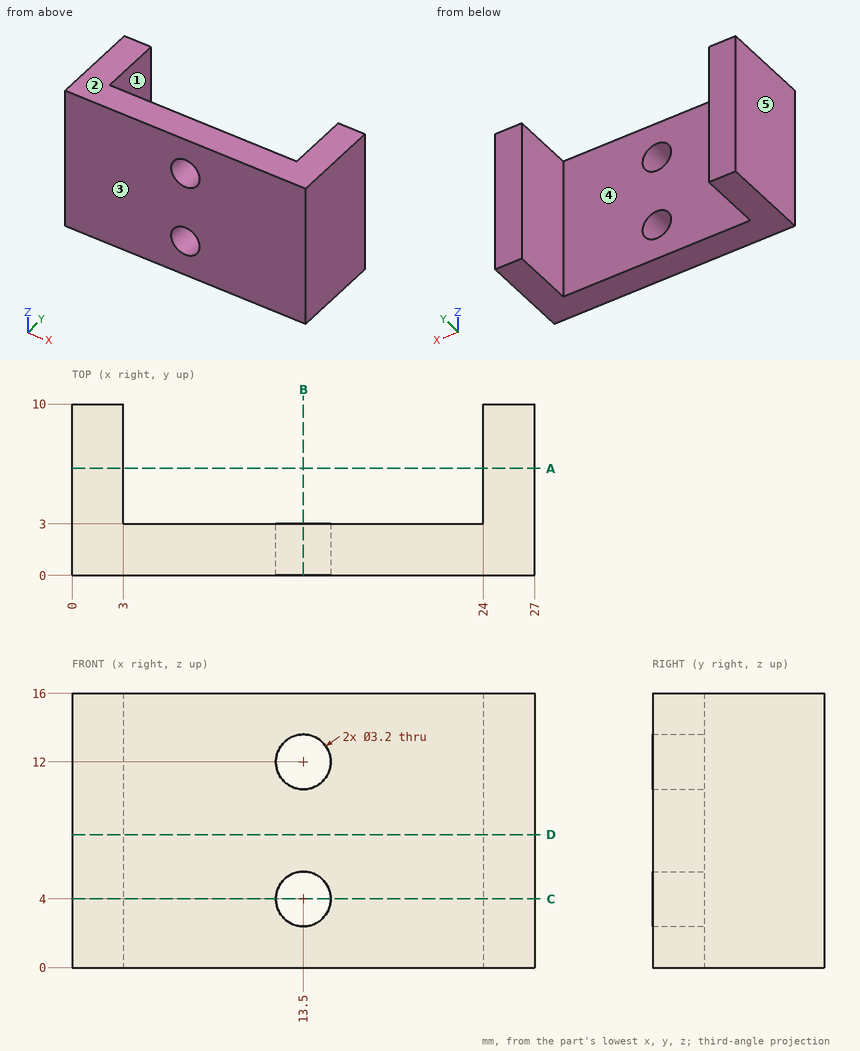
Job drawing, mm, ordinate dimensions from the low corner. One solid piece. A direction names the side the tool comes from. Round coordinates to 2 decimals unless told otherwise and drop trailing zeros. Order: outer loops, then holes, each group sorted by start corner. A loop starts at its lowest first (then second) coordinate and runs counter-clockwise, first axis right, second up. Notation, with made-up numbers: (76.5, 41) -> (132.5, 41) arc R33 ccw to (132.5, 80) -> close; hole circle Ø4 at (70, 31.25). An arc over 180 degrees is marked (long way). Answer in a Markdown table with one row per item.
1) Band-saw the part on A-A on y = 6.25. Give the cut face in (x, z), and give its area (3 significant figures).
Values:
| item | result |
|---|---|
| outline | (0, 0) -> (3, 0) -> (3, 16) -> (0, 16) -> close; (24, 0) -> (27, 0) -> (27, 16) -> (24, 16) -> close |
| area | 96.0 mm2 |
2) Mould opens along X. For the marked faces 3, 4 and 5 say: released by +X, released by -X, zero draft, split by the parting line, or undercut.
Values:
| item | result |
|---|---|
| face 3 | zero draft |
| face 4 | undercut |
| face 5 | released by -X |
3) Wall check: L1, parallel to Z at x = 13.5, y = 0.75; L2, parallel to X at y = 7.25, z = 7; L3, parallel to Y at x = 8, z = 1. Give the ranges that are in metal, low to high.
Values:
| item | result |
|---|---|
| L1 | 0 to 2.4, 5.6 to 10.4, 13.6 to 16 |
| L2 | 0 to 3, 24 to 27 |
| L3 | 0 to 3 |
4) Band-saw the part on D-D on z = 7.75. Give the cut face in (x, y).
Values:
| item | result |
|---|---|
| outline | (0, 0) -> (27, 0) -> (27, 10) -> (24, 10) -> (24, 3) -> (3, 3) -> (3, 10) -> (0, 10) -> close |
5) Pin check, flat tip, straight feed: P1, Ø5, axis at x = 13.5, z = 4, coming from the +Y side. Stop position of the tip, or through.
Values:
| item | result |
|---|---|
| P1 | y = 3 |
6) Band-saw the part on C-C on z = 4. Give the cut face in (x, y), and give its area (3 significant figures).
Values:
| item | result |
|---|---|
| outline | (0, 0) -> (11.9, 0) -> (11.9, 3) -> (3, 3) -> (3, 10) -> (0, 10) -> close; (15.1, 0) -> (27, 0) -> (27, 10) -> (24, 10) -> (24, 3) -> (15.1, 3) -> close |
| area | 113 mm2 |
7) Which spindle directions (+Z, -Z, +X, -X, +Y, -Y) get a long thin tool onto all of the face, cutting with end or side? Do the marked faces 1 and 2. Say none if no direction does.
Values:
| item | result |
|---|---|
| face 1 | +Z, -Z, +Y |
| face 2 | +Z, +X, -X, +Y, -Y |
8) Band-saw the part on B-B on x = 13.5. Give the cut face in (y, z), and give its area (3 significant figures).
Values:
| item | result |
|---|---|
| outline | (0, 0) -> (3, 0) -> (3, 2.4) -> (0, 2.4) -> close; (0, 5.6) -> (3, 5.6) -> (3, 10.4) -> (0, 10.4) -> close; (0, 13.6) -> (3, 13.6) -> (3, 16) -> (0, 16) -> close |
| area | 28.8 mm2 |
